```python
from build123d import *

# Parameters (mm, degrees)
SKETCH1_R          = 19.0373
BASE_EXTRUDE_DEPTH = 15.875


with BuildPart() as part:
    # Sketch1 → Base-Extrude (new, symmetric)
    with BuildSketch(Plane(origin=(0, 0, 0), x_dir=(0, 0, -1), z_dir=(1, 0, 0))):
        with BuildLine():
            Line((-38.090421481, 123.815421481), (-38.090421481, 47.615421481))
            ThreePointArc((-38.090421481, 47.615421481), (-40.880229391, 40.880229391), (-47.615421481, 38.090421481))
            Line((-47.615421481, 38.090421481), (-123.815421481, 38.090421481))
            Line((-123.815421481, 38.090421481), (-123.815421481, 34.182275097))
            ThreePointArc((-123.815421481, 34.182275097), (-122.495102851, 29.344007988), (-118.900181875, 25.847064595))
            Line((-118.900181875, 25.847064595), (-16.902454778, -30.562438507))
            ThreePointArc((-16.902454778, -30.562438507), (24.695704333, -24.695704333), (30.562438507, 16.902454778))
            Line((30.562438507, 16.902454778), (-25.847064595, 118.900181875))
            ThreePointArc((-25.847064595, 118.900181875), (-29.344007988, 122.495102851), (-34.182275097, 123.815421481))
            Line((-34.182275097, 123.815421481), (-38.090421481, 123.815421481))
        make_face()
        Circle(SKETCH1_R, mode=Mode.SUBTRACT)
    extrude(amount=BASE_EXTRUDE_DEPTH, both=True)


solid = part.part
```
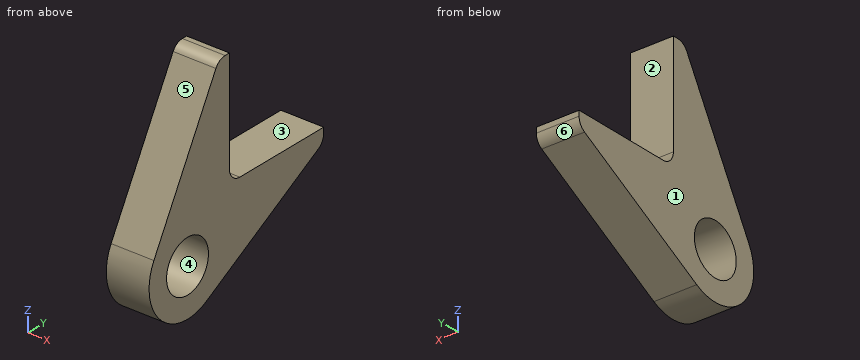
Input: part model. Units: mm. Frame: model coordinates. Face numbers are marked on the shaded views. A direction names the side the tool comes from. Round coordinates to 2 decimals unless told otherwise and drop trailing zeros. Loops run counter-clockwise (first coordinate to the right, second up) from the corner with the lowest first, then second, coordinate; pieces in that order, holes last. Notation, with made-up numbers: (-39.5, 41.25) -> (-25.5, 41.25) arc R21 ccw to (-25.5, 53.25) -> close; hole circle Ø10 at (43, 85.25). An arc over 180 degrees is marked (long way). Use one line per item in the form item = value. Start each with the question number.
Item 1: Section query D-D on z = 67. Return the cut outline in (x, y) (3 decimals).
Item 2: Section query A-A on x = 2.5. Return the cut outline in (y, z) (3 decimals).
Item 3: Material intervals for L1, parallel to Y at x = 0.5, z = 0 (3 decimals); L2, parallel to Z at x = 6, y = -15; L3, parallel to Z at x = 14, y = 100.5, sorted ascending. Write a range as from..to.
Item 4: Section query B-B on y = 11. Return the cut outline in (x, z) (3 decimals).
Item 5: Mould query, pull axis Y, two halves, no side actions, for the marked faces 3, 4, 5 and 6. Classes: pulls with the +Y half, pulls with the -Y half, needs draft (parallel to the pull), parting line crosses it, or undercut.
Item 6: Section query C-C on z = 0. Return the cut outline in (x, y) (3 decimals).
Item 7: Set-up query: the marked faces 1 and 2. Return all of +Z, -Z, +X, -X, +Y, -Y with unobstructed straight access to the full face (end or side cutting, diameter ignored); none if empty.
Item 8: Contact query for flat-ended pins moving along their axis: pin 1 Ø1.5 at (x, z) = (6, -15.5) entering from +Y; pin 2 Ø6 at (x, z) = (12.5, 75) entering from -Y; pin 3 Ø5 at (x, z) = (-8.5, 75) entering from +Y. Output: stop coordinate, or through.
Ans:
q1.outline = (-15.875, -2.856) -> (15.875, -2.856) -> (15.875, 38.09) -> (-15.875, 38.09) -> close
q2.outline = (-30.562, 16.902) arc R34.925 ccw to (16.902, -30.562) -> (118.9, 25.847) arc R9.525 ccw to (123.815, 34.182) -> (123.815, 38.09) -> (47.615, 38.09) arc R9.525 cw to (38.09, 47.615) -> (38.09, 123.815) -> (34.182, 123.815) arc R9.525 ccw to (25.847, 118.9) -> close; hole circle Ø38.075 at (0, 0)
q3.L1 = -34.925..-19.037, 19.037..72.164
q3.L2 = -31.54..-11.72, 11.72..45.04
q3.L3 = 15.67..38.09
q4.outline = (-15.875, -33.147) -> (15.875, -33.147) -> (15.875, -15.538) -> (-15.875, -15.538) -> close; (-15.875, 15.538) -> (15.875, 15.538) -> (15.875, 92.054) -> (-15.875, 92.054) -> close
q5.face_3 = needs draft
q5.face_4 = undercut
q5.face_5 = pulls with the -Y half
q5.face_6 = pulls with the +Y half
q6.outline = (-15.875, -34.925) -> (15.875, -34.925) -> (15.875, -19.037) -> (-15.875, -19.037) -> close; (-15.875, 19.037) -> (15.875, 19.037) -> (15.875, 72.164) -> (-15.875, 72.164) -> close
q7.face_1 = +Z, -Z, -X, +Y, -Y
q7.face_2 = +Z, +X, -X, +Y
q8.pin_1 = 45.49
q8.pin_2 = -0.09
q8.pin_3 = 38.09
